```python
from build123d import *

# Parameters (mm, degrees)
SKETCH1_R           = 203.2
SKETCH1_R_2         = 9.525
BOSS_EXTRUDE1_DEPTH = 6.35
BOSS_EXTRUDE2_DEPTH = 171.45
CIRPATTERN1_COUNT   = 3
SKETCH3_R           = 19.05
SKETCH3_R_2         = 9.525
BOSS_EXTRUDE3_DEPTH = 3.175


with BuildPart() as part:
    # Sketch1 → Boss-Extrude1 (new body)
    with BuildSketch(Plane.XY):
        Circle(SKETCH1_R)
        Circle(SKETCH1_R_2, mode=Mode.SUBTRACT)
    extrude(amount=BOSS_EXTRUDE1_DEPTH)

    # Sketch2 → Boss-Extrude2 (add)
    with BuildSketch(Plane(origin=(0, -25.4, 0), x_dir=(1, 0, 0), z_dir=(0, 1, 0))):
        Polygon((-4.7625, 0), (-4.7625, 76.2), (17.234545256, 88.9), (21.997045256, 80.651108029), (4.7625, 70.700738686), (4.7625, 0), align=None)
    boss_extrude2 = extrude(amount=-BOSS_EXTRUDE2_DEPTH)

    # CirPattern1: Boss-Extrude2 ×3 about axis
    cirpattern1_axis = Axis((0, 0, 0), (0, 0, 1))
    for i in range(1, CIRPATTERN1_COUNT):
        add(boss_extrude2.rotate(cirpattern1_axis, i * 360 / CIRPATTERN1_COUNT))

    # Sketch3 → Boss-Extrude3 (add)
    with BuildSketch(Plane.XY.offset(6.35)):
        Circle(SKETCH3_R)
        Circle(SKETCH3_R_2, mode=Mode.SUBTRACT)
    extrude(amount=BOSS_EXTRUDE3_DEPTH)


solid = part.part
```
Here's how the part is built. I have some questions about the finished solid (model axes, mm). A direction names the side the tool comes from. Round coordinates to 2 decimals unless told otherwise and drop trailing zeros. Order: outer loops, then holes, each group sorted by start corner. A loop starts at its lowest first (then second) coordinate and runs counter-clockwise, first axis right, second up. Notation, with made-up numbers: M -3.5,-32 L 52.5,-32 A22 ccw 52.5,-10 Z; hole C 35.5,73.5 d8. An arc over 180 degrees is marked long. Use CSV: the item, a comma, the result in double quotes.
1) I want a section at B-B (x = 0). List the corners of the cut face in (y, z) for me (3 decimals), then the cut area to 3 significant figures.
Taken from the geometry:
outline,"M -203.2,0 L -196.85,0 L -196.85,-78.95 L -25.4,-78.95 L -25.4,0 L -9.525,0 L -9.525,9.525 L -19.05,9.525 L -19.05,6.35 L -203.2,6.35 Z; M 9.525,0 L 203.2,0 L 203.2,6.35 L 19.05,6.35 L 19.05,9.525 L 9.525,9.525 Z"
area,"16,100 mm^2"
2) I want a section at A-A (z = -29). List the corners of the cut face in (x, y) for me, then the cut area to 3 significant figures.
Taken from the geometry:
outline,"M -172.86,94.3 L -24.38,8.58 L -19.62,16.82 L -168.1,102.55 Z; M -4.76,-196.85 L 4.76,-196.85 L 4.76,-25.4 L -4.76,-25.4 Z; M 19.62,16.82 L 24.38,8.58 L 172.86,94.3 L 168.1,102.55 Z"
area,"4,900 mm^2"
3) I want a section at D-D (x = -159). List the corners of the cut face in (y, z) for me, then the cut area to 3 significant figures.
Taken from the geometry:
outline,"M -126.53,0 L 86.3,0 L 86.3,-70.7 L 66.4,-80.65 L 71.9,-88.9 L 97.3,-76.2 L 97.3,0 L 126.53,0 L 126.53,6.35 L -126.53,6.35 Z"
area,"2,660 mm^2"
4) On a 3-axis mill with a long thin cutter (end or side, diameter ignored), from which of +Z, -Z, +X, -X, +Y, -Y can I reach the whole of each face in a straight line? I mean faces 1 (the flat face through (-171.844, 96.058, -47.95)), 2 (the flat face through (169.11, 100.79, -47.95)), 3 (the flat face through (-23.364, 10.333, -47.95)), 4 (the flat face through (-97.58, 50.84, -35.85)). Say none if no direction works.
Taken from the geometry:
face 1,"-Z, -X, +Y"
face 2,"-Z, +X, +Y"
face 3,"-Z, -Y"
face 4,"-X, -Y"
5) I'm going to push flat-ended pins straight in: P1, Ø5, axis at y = -110.5, z = -26, coming from the +X side; P2, Ø2, axis at x = -80, z = -71, coming from the -Y side; P3, Ø12, axis at x = -115, z = -35, coming from the +Y side. Where does each tip first touch, or does it pass through?
Taken from the geometry:
P1,"x = 4.76"
P2,"y = 38.01"
P3,"y = 75.36"
6) I want a section at C-C (y = -82.5). List the corners of the cut face in (x, z) for me, then the cut area to 3 significant figures.
Taken from the geometry:
outline,"M -185.7,0 L -4.76,0 L -4.76,-76.2 L 17.23,-88.9 L 22,-80.65 L 4.76,-70.7 L 4.76,0 L 185.7,0 L 185.7,6.35 L -185.7,6.35 Z"
area,"3,270 mm^2"
7) If we mould it in two halves opening along X, with no side actions, what happens to faces 5 (the flat face through (88.448, 66.654, -75.746)), 6 (the flat face through (6.08, -109.92, -82.46)), 7 (the cylindrical face through (-15.12, -11.59, 7.92))? For each: pulls with the +X half, pulls with the -X half, needs draft (parallel to the pull), parting line crosses it, or undercut.
Taken from the geometry:
face 5,"undercut"
face 6,"pulls with the -X half"
face 7,"parting line crosses it"
8) I need wall thicknesses on line 1 along Y through (x, z) = (0, 3.75) (3 decimals); line 2 along Z through (x, y) = (-72, 121.5); line 3 along X through (y, z) = (-126, -67). Which ranges of each line are inside material? Lowest first, please. Write a range as [from, to].
Taken from the geometry:
line 1,"[-203.2, -9.525], [9.525, 203.2]"
line 2,"[0, 6.35]"
line 3,"[-4.76, 4.76]"
